Verification items for the finished model (mm, model axes). Face numbers are marked on the shaded views. A direction names the side the tool comes from. Give positions to 0.01 mm unless a question says otherwise; leave off trailing zeros. Write each loop counter-clockwise with the first axis right and the second up, starting at its lowest first coordinate (ties: lowest second). Pieces come first, ordered by that corner, then holes. Notation, with made-up numbers: (-1.5, -3) -> (49.5, -3) arc R23 ccw to (49.5, 33) -> close; hole circle Ø2 at (10, -19). An arc over 180 degrees is marked (long way). Answer as CSV lines item,"result".
```python
from build123d import *

# Parameters (mm, degrees)
EXTRUDE_2_DEPTH     = 108
CHAMFER_2_SIZE      = 4
SKETCH_3_R          = 42.5
CUT_EXTRUDE_1_DEPTH = 166.024240644
SKETCH_4_R          = 45
CUT_EXTRUDE_2_DEPTH = 11
CUT_EXTRUDE_START   = -11
SKETCH_5_R          = 45
CUT_EXTRUDE_3_DEPTH = 11
SKETCH_6_R          = 5
CUT_EXTRUDE_4_DEPTH = 21
SKETCH_10_R         = 47.5
CUT_EXTRUDE_5_DEPTH = 2
SKETCH_11_R         = 42.5
CUT_EXTRUDE_6_DEPTH = 55


with BuildPart() as part:
    # 草图2 → 凸台-拉伸2 (new body)
    with BuildSketch(Plane(origin=(0, 0, 0), x_dir=(1, 0, 0), z_dir=(0, 1, 0))):
        with BuildLine():
            Line((-50, 0), (50, 0))
            Line((50, 0), (55, 55))
            Line((55, 55), (55, 57))
            ThreePointArc((55, 57), (0, 112), (-55, 57))
            Line((-55, 57), (-55, 55))
            Line((-55, 55), (-50, 0))
        make_face()
    extrude(amount=EXTRUDE_2_DEPTH)

    # 倒角2
    # the kernel refuses this chamfer: 4 mm, written as the material it takes off along each edge
    with BuildSketch(Plane(origin=(-55.931316952, 108, -65.244486468), x_dir=(-0.02738295672235633, -0.9996219169112968, 0.00248935970203239), z_dir=(0.0905357460425184, 0, 0.9958932064677039)), Plane(origin=(49.068683048, 108, 10.244486468), x_dir=(0.027382956722356445, -0.9996219169112968, 0.0024893597020324005), z_dir=(0.0905357460425184, 0, -0.9958932064677039))) as chamfer_2_piece_1:
        Polygon((CHAMFER_2_SIZE * 0.999621916911, CHAMFER_2_SIZE * 0.0274958766106), (-CHAMFER_2_SIZE * 0.0274958766106, CHAMFER_2_SIZE * 0.999621916911), (0, 0), align=None)
    extrude(amount=75.80026899, mode=Mode.SUBTRACT)
    with BuildSketch(Plane(origin=(-60.286731952, 108, 0), x_dir=(0, -0.9996219169112968, 0.02749587661058639), z_dir=(1, 0, 0))) as chamfer_2_piece_2:
        Polygon((CHAMFER_2_SIZE * 0.999621916911, CHAMFER_2_SIZE * 0.0274958766106), (-CHAMFER_2_SIZE * 0.0274958766106, CHAMFER_2_SIZE * 0.999621916911), (0, 0), align=None)
    extrude(amount=120.573463904, mode=Mode.SUBTRACT)
    with BuildSketch(Plane(origin=(55, 108, -44.713268048), x_dir=(0.027495876610585647, -0.9996219169112968, 0), z_dir=(0, 0, -1)), Plane(origin=(-55, 108, -57), x_dir=(-0.027495876610585647, -0.9996219169112968, 0), z_dir=(0, 0, 1))) as chamfer_2_piece_3:
        Polygon((CHAMFER_2_SIZE * 0.999621916911, CHAMFER_2_SIZE * 0.0274958766106), (-CHAMFER_2_SIZE * 0.0274958766106, CHAMFER_2_SIZE * 0.999621916911), (0, 0), align=None)
    extrude(amount=12.286731952, mode=Mode.SUBTRACT)
    with BuildSketch(Plane(origin=(0, 108, -57), x_dir=(1, 0, 0), z_dir=(0, 0, 1))) as chamfer_2_piece_4:
        Polygon((55, -CHAMFER_2_SIZE), (55 - CHAMFER_2_SIZE, 0), (55, 0), align=None)
    revolve(axis=Axis((0, 108, -57), (0, 1, 0)), revolution_arc=180, mode=Mode.SUBTRACT)
    with BuildSketch(Plane(origin=(55, 0, -44.713268048), x_dir=(0.02749587661058563, 0.9996219169112968, 0), z_dir=(0, 0, -1)), Plane(origin=(-55, 0, -57), x_dir=(-0.02749587661058563, 0.9996219169112968, 0), z_dir=(0, 0, 1))) as chamfer_2_piece_5:
        Polygon((CHAMFER_2_SIZE * 0.999621916911, -CHAMFER_2_SIZE * 0.0274958766106), (-CHAMFER_2_SIZE * 0.0274958766106, -CHAMFER_2_SIZE * 0.999621916911), (0, 0), align=None)
    extrude(amount=12.286731952, mode=Mode.SUBTRACT)
    with BuildSketch(Plane(origin=(49.068683048, 0, 10.244486468), x_dir=(0.027382956722356428, 0.9996219169112968, 0.0024893597020323992), z_dir=(0.0905357460425184, 0, -0.9958932064677039)), Plane(origin=(-55.931316952, 0, -65.244486468), x_dir=(-0.027382956722356314, 0.9996219169112968, 0.0024893597020323884), z_dir=(0.0905357460425184, 0, 0.9958932064677039))) as chamfer_2_piece_6:
        Polygon((CHAMFER_2_SIZE * 0.999621916911, -CHAMFER_2_SIZE * 0.0274958766106), (-CHAMFER_2_SIZE * 0.0274958766106, -CHAMFER_2_SIZE * 0.999621916911), (0, 0), align=None)
    extrude(amount=75.80026899, mode=Mode.SUBTRACT)
    with BuildSketch(Plane(origin=(-60.286731952, 0, 0), x_dir=(0, 0.9996219169112968, 0.027495876610586372), z_dir=(1, 0, 0))) as chamfer_2_piece_7:
        Polygon((CHAMFER_2_SIZE * 0.999621916911, -CHAMFER_2_SIZE * 0.0274958766106), (-CHAMFER_2_SIZE * 0.0274958766106, -CHAMFER_2_SIZE * 0.999621916911), (0, 0), align=None)
    extrude(amount=120.573463904, mode=Mode.SUBTRACT)
    with BuildSketch(Plane(origin=(0, 0, -57), x_dir=(1, 0, 0), z_dir=(0, 0, 1))) as chamfer_2_piece_8:
        Polygon((55, CHAMFER_2_SIZE), (55 - CHAMFER_2_SIZE, 0), (55, 0), align=None)
    revolve(axis=Axis((0, 0, -57), (0, 1, 0)), revolution_arc=180, mode=Mode.SUBTRACT)

    # 草图3 → 切除-拉伸1 (cut, through all)
    with BuildSketch(Plane(origin=(0, 108, 0), x_dir=(1, 0, 0), z_dir=(0, 1, 0))):
        with Locations(Location((0, 57, 0), (0, 0, 270))):
            Circle(SKETCH_3_R)
    extrude(amount=-CUT_EXTRUDE_1_DEPTH, mode=Mode.SUBTRACT)

    # 草图4 → 切除-拉伸2 (cut)
    with BuildSketch(Plane(origin=(0, 108, 0), x_dir=(1, 0, 0), z_dir=(0, 1, 0))):
        with Locations(Location((0, 57, 0), (0, 0, 270))):
            Circle(SKETCH_4_R)
    extrude(amount=-CUT_EXTRUDE_2_DEPTH, mode=Mode.SUBTRACT)

    # 草图5 → 切除-拉伸3 (cut)
    with BuildSketch(Plane.XZ.offset(CUT_EXTRUDE_START)):
        with Locations(Location((0, -57, 0), (0, 0, 90))):
            Circle(SKETCH_5_R)
    extrude(amount=CUT_EXTRUDE_3_DEPTH, mode=Mode.SUBTRACT)

    # 草图6 → 切除-拉伸4 (cut)
    with BuildSketch(Plane.XY):
        with Locations((40, 94)):
            Circle(SKETCH_6_R)
        with Locations((-40, 94)):
            Circle(SKETCH_6_R)
        with Locations((-40, 14)):
            Circle(SKETCH_6_R)
        with Locations((40, 14)):
            Circle(SKETCH_6_R)
    extrude(amount=-CUT_EXTRUDE_4_DEPTH, mode=Mode.SUBTRACT)

    # 草图8 → 切除-旋转2 (revolve, cut)
    with BuildSketch(Plane(origin=(0, 89, 0), x_dir=(1, 0, 0), z_dir=(0, 1, 0)), mode=Mode.PRIVATE) as cut_revolve_2_sk:
        Polygon((55, 57), (25, 57), (25, 55), (45, 55), (45, 52), (55, 52), align=None)
    revolve(cut_revolve_2_sk.sketch.rotate(Axis((51, 89, -57), (-1, 0, 0)), 180), axis=Axis((51, 89, -57), (-1, 0, 0)), mode=Mode.SUBTRACT)

    # 草图9 → 切除-旋转3 (revolve, cut)
    with BuildSketch(Plane(origin=(0, 69, 0), x_dir=(1, 0, 0), z_dir=(0, 1, 0)), mode=Mode.PRIVATE) as cut_revolve_3_sk:
        Polygon((55, 57), (25, 57), (25, 55), (45, 55), (45, 52), (55, 52), align=None)
    revolve(cut_revolve_3_sk.sketch.rotate(Axis((55, 69, -57), (-1, 0, 0)), 180), axis=Axis((55, 69, -57), (-1, 0, 0)), mode=Mode.SUBTRACT)

    # 草图10 → 切除-拉伸5 (cut)
    with BuildSketch(Plane.XY):
        with Locations((0, 54)):
            Circle(SKETCH_10_R)
    extrude(amount=-CUT_EXTRUDE_5_DEPTH, mode=Mode.SUBTRACT)

    # 草图11 → 切除-拉伸6 (cut)
    with BuildSketch(Plane.XY.offset(-2)):
        with Locations((0, 54)):
            Circle(SKETCH_11_R)
    extrude(amount=-CUT_EXTRUDE_6_DEPTH, mode=Mode.SUBTRACT)


solid = part.part
```
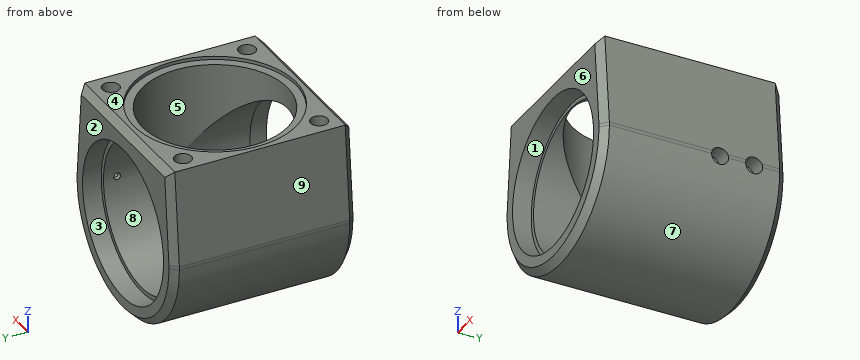
1) Scan lines: line 1 along Y through (x, z) = (-0.5, -7); line 2 along Y through (x, z) = (44.3, -57); line 3 along Y through (x, z) = (-36.5, -11). Record each from-to range of solid material in increasing order.
Reported:
line 1,"0 to 11.5, 96.5 to 108"
line 2,"11 to 67, 71 to 87, 91 to 97"
line 3,"0 to 10.43, 17.57 to 32.23, 75.77 to 90.43, 97.57 to 108"
2) Section check B-B (y = 69). Record the boundary of the cut face in (x, z), and give its area (3 significant figures).
Reported:
outline,"(-55, -57) arc R55 ccw to (54.77, -62) -> (45, -62) -> (45, -59) -> (42.45, -59) arc R42.5 cw (long way) to (-39.76, -42) -> (-39.76, -2) -> (-45.07, -2) -> (-45.07, 0) -> (-50, 0) -> (-55, -55) -> close; (39.76, -42) arc R42.5 cw to (42.45, -55) -> (45, -55) -> (45, -52) -> (54.73, -52) -> (50, 0) -> (45.07, 0) -> (45.07, -2) -> (39.76, -2) -> close"
area,"3,190 mm²"
3) Tool access check on the marked faces 1, 2, 3, 4 and 5. Record the directions out of +Z, -Z, +X, -X, +Y, -Y that give a thin tool (end or side, any length) a straight path to the whole face; none if there is none.
Reported:
face 1,"-Y"
face 2,"+Z, -Z, +X, -X, +Y"
face 3,"+Y"
face 4,"+Z, +X, -X, +Y, -Y"
face 5,"+Z"
4) Depth check by flat-ended pin: pin 1 (1 mm diameter, centred on y = 15, z = -86.5, fed in from +X); pin 2 (10 mm diameter, centred on x = 38, y = 46, fed in from -Z); pin 3 (2 mm diameter, centred on x = -39, z = -38.5, fed in from -Y). Enter the tip coordinate at first touch or a pass-through.
Reported:
pin 1,"x = 46.73"
pin 2,"z = -101"
pin 3,"y = 11"
5) Draft check along X on the marked faces 6, 7, 8 and 9. Enter one of: +X half, -X half, draft (parallel to the pull), parting line (faces both ways), or undercut.
Reported:
face 6,"draft"
face 7,"parting line"
face 8,"undercut"
face 9,"-X half"
6) Section check A-A (x = 0). Record the boundary of the cut face in (y, z).
Reported:
outline,"(0, -108) -> (4, -112) -> (104, -112) -> (108, -108) -> (108, -102) -> (97, -102) -> (97, -99.5) -> (11, -99.5) -> (11, -102) -> (0, -102) -> close; (0, -12) -> (11, -12) -> (11, -14.5) -> (11.5, -14.5) -> (11.5, -2) -> (6.5, -2) -> (6.5, 0) -> (4, 0) -> (0, -4) -> close; (96.5, -14.5) -> (97, -14.5) -> (97, -12) -> (108, -12) -> (108, -4) -> (104, 0) -> (101.5, 0) -> (101.5, -2) -> (96.5, -2) -> close"
7) Section check C-C (z = -43.5). Record the boundary of the cut face in (x, y).
Reported:
outline,"(-53.95, 4) -> (-49.94, 0) -> (-42.93, 0) -> (-42.93, 11) -> (-40.3, 11) -> (-40.3, 40.5) arc R42.5 cw to (-40.3, 67.5) -> (-40.3, 97) -> (-42.93, 97) -> (-42.93, 108) -> (-49.94, 108) -> (-53.95, 104) -> close; (40.3, 11) -> (42.93, 11) -> (42.93, 0) -> (49.94, 0) -> (53.95, 4) -> (53.95, 104) -> (49.94, 108) -> (42.93, 108) -> (42.93, 97) -> (40.3, 97) -> (40.3, 67.5) arc R42.5 cw to (40.3, 40.5) -> close"
8) Section check D-D (y = 16). Record the boundary of the cut face in (x, z).
Reported:
outline,"(-55, -57) arc R55 ccw to (55, -57) -> (55, -55) -> (50, 0) -> (44.58, 0) -> (44.58, -21) -> (35.42, -21) -> (35.42, 0) -> (28.5, 0) -> (28.5, -2) -> (19.03, -2) -> (19.03, -19) arc R42.5 cw (long way) to (-19.03, -19) -> (-19.03, -2) -> (-28.5, -2) -> (-28.5, 0) -> (-35.42, 0) -> (-35.42, -21) -> (-44.58, -21) -> (-44.58, 0) -> (-50, 0) -> (-55, -55) -> close"
